from build123d import *

# Parameters (mm, degrees)
SKETCH029_W  = 14
SKETCH029_H  = 14
PAD014_DEPTH = 10
SKETCH030_R  = 3.5
PAD015_DEPTH = 7
SKETCH031_R  = 3
PAD016_DEPTH = 15


with BuildPart() as part:
    # Sketch029 → Pad014 (new body)
    with BuildSketch(Plane.XY):
        with Locations((7, 7)):
            Rectangle(SKETCH029_W, SKETCH029_H)
    extrude(amount=-PAD014_DEPTH)

    # Sketch030 → Pad015 (join)
    with BuildSketch(Plane.XY):
        with Locations((7, 7)):
            Circle(SKETCH030_R)
    extrude(amount=PAD015_DEPTH)

    # Sketch031 (on Face8 of Pad015) → Pad016 (join)
    with BuildSketch(Plane.XY.offset(7)):
        with Locations((7, 7)):
            Circle(SKETCH031_R)
    extrude(amount=PAD016_DEPTH)


with BuildPart() as part_1:
    # Body004 placement: moved
    add(part.part.moved(Location((11, 47, 39.4))))


solid = part_1.part
Model file for the job. Use its own axes, mm. A direction names the side the tool comes from. Give positions to 0.01 mm unless a question says otherwise; leave off trailing zeros. Loops run counter-clockwise (first coordinate to the right, second up) from the corner with the lowest first, then second, coordinate; pieces in that order, holes last. Notation, with made-up numbers: (75, 47.5) -> (94, 47.5) arc R25 ccw to (94, 74.5) -> close; hole circle Ø10 at (87.25, -39). An arc over 180 degrees is marked (long way). Use a Markdown table: item, result. Add a question column.
(1) Slice it at A-A on y = 54. List the corners of the cut face in (x, z).
(2) Tool access for faces 1 (the flat face through (18, 61, 34)), 2 (the flat face through (15, 57, 39.4)): list every direction of +Z, -Z, +X, -X, +Y, -Y with a clear straight run to the whole face (end or side of a thin tool).
(3) Slice it at B-B on x = 18. List the corners of the cut face in (y, z).
(4) Slice it at C-C on z = 45.5. List the corners of the cut face in (x, y), and give its area (3 significant figures).
(5) Slice it at D-D on y = 49. List the corners of the cut face in (x, z).
(6) Drop flat-ended pins along their axis: pin 1 Ø8 at (y, z) = (56.5, 57.5) entering from +X; pin 2 Ø4 at (y, z) = (49.5, 51.5) entering from -X; pin 3 Ø6 at (x, z) = (18.5, 55.5) entering from +Y. Give the stop position or say it passes through.
(7) Wall check: line 1 along Z through (x, y) = (17.25, 50); line 2 along Z through (x, y) = (17.25, 57.25); line 3 along X through (y, z) = (55.5, 39.5). Give the ranges that are in metal, low to high.
Filled sheet:
| question | item | result |
|---|---|---|
| 1 | outline | (11, 29.4) -> (25, 29.4) -> (25, 39.4) -> (21.5, 39.4) -> (21.5, 46.4) -> (21, 46.4) -> (21, 61.4) -> (15, 61.4) -> (15, 46.4) -> (14.5, 46.4) -> (14.5, 39.4) -> (11, 39.4) -> close |
| 2 | face 1 | +Z, -Z, +X, -X, +Y |
| 2 | face 2 | +Z |
| 3 | outline | (47, 29.4) -> (61, 29.4) -> (61, 39.4) -> (57.5, 39.4) -> (57.5, 46.4) -> (57, 46.4) -> (57, 61.4) -> (51, 61.4) -> (51, 46.4) -> (50.5, 46.4) -> (50.5, 39.4) -> (47, 39.4) -> close |
| 4 | outline | circle Ø7 at (18, 54) |
| 4 | area | 38.5 mm2 |
| 5 | outline | (11, 29.4) -> (25, 29.4) -> (25, 39.4) -> (11, 39.4) -> close |
| 6 | pin 1 | x = 21 |
| 6 | pin 2 | x = 16.34 |
| 6 | pin 3 | y = 57 |
| 7 | line 1 | 29.4 to 39.4 |
| 7 | line 2 | 29.4 to 46.4 |
| 7 | line 3 | 14.84 to 21.16 |
